Autodesk Inventor part; units mm, degrees
ref_plane "YZ Plane" through (0, 0, 0) normal (1, 0, 0) x (0, 1, 0)
ref_plane "XZ Plane" through (0, 0, 0) normal (0, 1, 0) x (-1, 0, 0)
ref_plane "XY Plane" through (0, 0, 0) normal (0, 0, 1) x (1, 0, 0)
sketch "Sketch1" plane through (0, 0, 0) normal (0, 0, 1) x (1, 0, 0)
  line L0 (-6.35, -3.6662) -> (-6.35, 3.6662)
  line L1 (-6.35, 3.6662) -> (0, 7.3323)
  line L2 (0, 7.3323) -> (6.35, 3.6662)
  line L3 (6.35, 3.6662) -> (6.35, -3.6662)
  line L4 (6.35, -3.6662) -> (0, -7.3323)
  line L5 (0, -7.3323) -> (-6.35, -3.6662)
  point P0 (0, 0)
  point P1 (0, 0)
  dimension "d0" = 12.7
extrude "Extrusion1" add sketch "Sketch1" along normal blind 70.1802
sketch "Sketch2" plane through (0, 0, 70.1802) normal (0, 0, 1) x (1, 0, 0)
  point P0 (0, 0)
  point P1 (0, 0)
hole "Hole1" at (0, 0, 70.1802) direction (0, 0, -1) diameter 3.9624 depth 13.6144 tip angle 118
sketch "Sketch3" plane through (0, 0, 0) normal (0, 0, -1) x (-1, 0, 0)
  circle A0 centre (0, 0) radius 1.9812
hole "Hole2" at (0, 0, 0) direction (0, 0, 1) diameter 3.9624 depth 13.6144 tip angle 118
properties part number "STOCK,HEX,SHAFT,TURRET,DRIVE" material "Aluminum 6061"
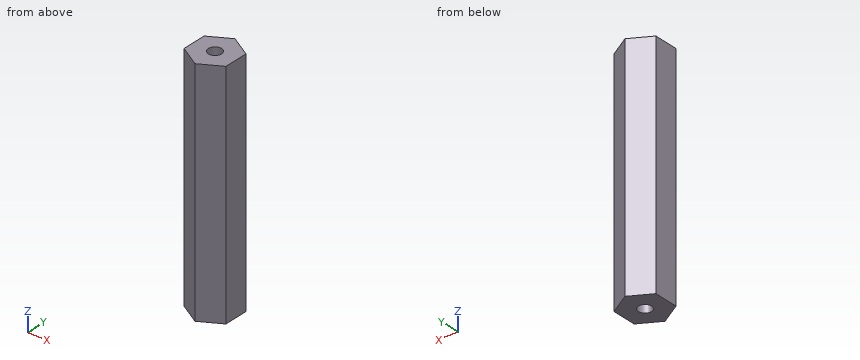
Check sheet for the modelled part. Datum: model origin and axes. Units: mm. Coordinates: 2 decimals unless noted, no trailing zeros. Loops run counter-clockwise (first coordinate to the right, second up) from the corner with the lowest first, then second, coordinate; pieces in that order, holes last. Notation, with made-up numbers: M 56,6 L 107,6 A27 ccw 107,43 Z; hole C -29,44.25 d4. An arc over 180 degrees is marked long. Answer as a JSON object with one key per item and string values.
1. Sectioned sample at B-B on y = -5.25. Record the cut outline in (x, z), and give its area (3 significant figures).
Outcome:
{"outline": "M -3.61,0 L 3.61,0 L 3.61,70.18 L -3.61,70.18 Z", "area": "506 mm²"}
2. Scan lines: L1, parallel to Y at x = 0, z = 60.75; L2, parallel to X at y = 0, z = 7.5; L3, parallel to Y at x = -5, z = 29. Record each from-to range of solid material in increasing order. Write a range as from..to.
Outcome:
{"L1": "-7.33..-1.98, 1.98..7.33", "L2": "-6.35..-1.98, 1.98..6.35", "L3": "-4.45..4.45"}
3. Sectioned sample at C-C on x = 5. Record the cut outline in (y, z), and give its area (3 significant figures).
Outcome:
{"outline": "M -4.45,0 L 4.45,0 L 4.45,70.18 L -4.45,70.18 Z", "area": "624 mm²"}
4. Sectioned sample at A-A on z = 31.5. Record the cut outline in (x, y).
Outcome:
{"outline": "M -6.35,-3.67 L 0,-7.33 L 6.35,-3.67 L 6.35,3.67 L 0,7.33 L -6.35,3.67 Z"}
5. Depth check by flat-ended pin: P1, Ø3.5, axis at x = 0, y = 0, coming from the -Z side; P2, Ø1.5, axis at x = 2.5, z = 7.5, coming from the -Y side; P3, Ø1.5, axis at x = -2, z = 55.5, coming from the +Y side. Enter the tip coordinate at first touch or a pass-through.
Outcome:
{"P1": "z = 13.75", "P2": "y = -6.32", "P3": "y = 6.61"}
